Read the model definition and answer for the solid it produces. Units are mm, in the model's axes. Face numbers are marked on the shaded views. A direction names the side the tool comes from. Coordinates: 2 decimals unless noted, no trailing zeros. Write each loop counter-clockwise with the first axis right and the second up, starting at its lowest first coordinate (ties: lowest second). Pieces come first, ordered by that corner, then holes.
1) Determine the mould class of the marked faces 5, 6 and 7 for opening direction X: +X half, -X half, draft (parallel to the pull), parting line (faces both ways), or undercut.
2) Which of the six approach directions +Z, -Z, +X, -X, +Y, -Y give full straight-line access (tool end or side, diameter ignored) to the marked faces 1, 2, 3 and 4?
3) Each of these flat-tipped pins is pushed along its axis until it touches: pin 1 Ø5.5 at (x, z) = (-25.5, 12.5) entering from -Y; pin 2 Ø22.5 at (y, z) = (-8, 47) entering from -X; pin 3 Ø11.5 at (x, y) = (4.5, -1) entering from +Z; pin 4 Ø2 at (x, y) = (-9, 11) entering from -Z. Where does it stop, or does it pass through?
4) The part is cut by section C-C (z = 41.5). Determine the outline of the cut face in (x, y).
5) Find the intervals of material crossed by line 1 (X direction, y = 0, z = 6.25); line 2 (X direction, y = 7, z = 54); line 3 (Y direction, x = -57, z = 11), in increasing order.
6) The part is cut by section A-A (x = -57). Determine the outline of the cut face in (y, z), then the cut area to 3 significant figures.
7) The part is cut by section B-B (y = 0). Determine the outline of the cut face in (x, z), then the cut area to 3 significant figures.
8) The part is cut by section D-D (y = 25). Determine the outline of the cut face in (x, z), then the cut area to 3 significant figures.
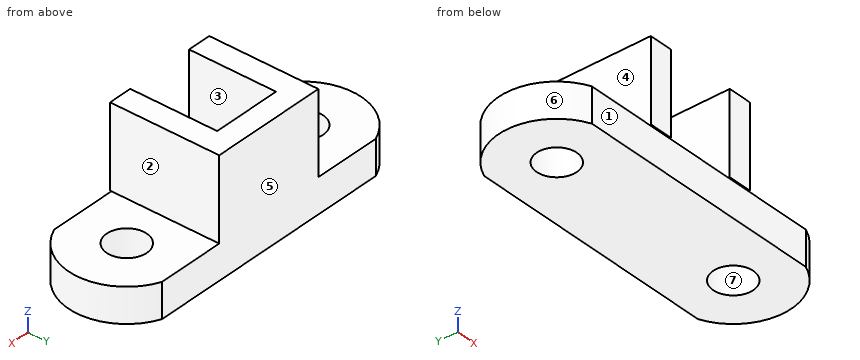
Autodesk Fusion 360 part; units mm, degrees
sketch "Sketch2" plane through (0, 0, 0) normal (0, 0, 1) x (1, 0, 0)
  line L0 (57, 29.6362) -> (-57, 29.6362)
  line L1 (-57, 29.6362) -> (-57, -29.6362)
  line L2 (-57, -29.6362) -> (57, -29.6362)
  line L3 (57, -29.6362) -> (57, 29.6362)
  line L4 (57, 29.6362) -> (-57, -29.6362) construction
  line L5 (-57, 29.6362) -> (57, -29.6362) construction
  circle A0 centre (57, 0) radius 11
  circle A1 centre (-57, 0) radius 11
  line L6 (57, 29.6362) -> (69.0705, 29.6362)
  line L7 (57, -29.6362) -> (69.0705, -29.6362)
  line L8 (69.0705, 29.6362) -> (69.0705, -29.6362)
  line L9 (-57, -29.6362) -> (-69.0705, -29.6362)
  line L10 (-57, 29.6362) -> (-69.0705, 29.6362)
  line L11 (-69.0705, 29.6362) -> (-69.0705, -29.6362)
  arc A2 (-69.0705, 29.6362) -> (-69.0705, -29.6362) centre (-57, 0) ccw
  arc A3 (69.0705, -29.6362) -> (69.0705, 29.6362) centre (57, 0) ccw
  dimension "d1" = 114
  dimension "d2" = 59.2723
  dimension "d3" = 22
  dimension "d4" = 22
  dimension "d5" = 64
  dimension "d6" = 64
extrude "Extrude1" add sketch "Sketch2" along normal blind 19 contours L0 L1 L2 L3 A0 A1 | L3 A0 L6 L7 L8 | L1 A1 L9 L10 L11 | L8 A3 | L11 A2
sketch "Sketch3" plane through (0, 0, 19) normal (0, 0, 1) x (-1, 0, 0)
  circle A0 centre (57, 0) radius 11
  circle A1 centre (-57, 0) radius 11
  line L0 (69.0705, 29.6362) -> (-69.0705, 29.6362)
  arc A2 (-69.0705, 29.6362) -> (-69.0705, -29.6362) centre (-57, 0) ccw
  line L1 (-69.0705, -29.6362) -> (69.0705, -29.6362)
  arc A3 (69.0705, -29.6362) -> (69.0705, 29.6362) centre (57, 0) ccw
  line L2 (32, -29.6362) -> (32, 29.6362) construction
  line L3 (-32, -29.6362) -> (-32, 29.6362) construction
  dimension "d9" = 64
  dimension "d10" = 25
sketch "Sketch4" plane through (0, 29.6362, 0) normal (0, 1, 0) x (-1, 0, 0)
  line L0 (-69.0705, 0) -> (69.0705, 0)
  line L1 (69.0705, 0) -> (69.0705, 19)
  line L2 (69.0705, 19) -> (-69.0705, 19)
  line L3 (-69.0705, 19) -> (-69.0705, 0)
  line L4 (-32.0857, 19) -> (31.9143, 19)
  line L5 (31.9143, 19) -> (31.9143, 64)
  line L6 (31.9143, 64) -> (-32.0857, 64)
  line L7 (-32.0857, 64) -> (-32.0857, 19)
  dimension "d11" = 64
  dimension "d12" = 45
extrude "Extrude2" add sketch "Sketch4" against normal blind 60 contours L2 L4 L5 L6 L7
sketch "Sketch5" plane through (0, 0, 64) normal (0, 0, 1) x (-1, 0, 0)
  line L0 (-32.0857, -29.6362) -> (31.9143, -29.6362)
  line L1 (31.9143, -29.6362) -> (31.9143, 30.3638)
  line L2 (31.9143, 30.3638) -> (-32.0857, 30.3638)
  line L3 (-32.0857, 30.3638) -> (-32.0857, -29.6362)
  line L4 (31.9143, -17.4462) -> (-32.0857, -17.4462)
  line L5 (18.9143, -17.4462) -> (18.9143, 30.3638)
  line L6 (-19.0857, -17.4462) -> (-19.0857, 30.3638)
  dimension "d15" = 12.19
  dimension "d16" = 38
  dimension "d17" = 13
extrude "Extrude3" cut sketch "Sketch5" against normal blind 45 contours L2 L4 L5 L6
equation "d12 = 64 mm - 19 mm"
Reported:
1. face 5: draft
1. face 6: -X half
1. face 7: undercut
2. face 1: -Z, +X, -X, -Y
2. face 2: +Z, +X, +Y, -Y
2. face 3: +Z, -Y
2. face 4: +Z, -X, +Y, -Y
3. pin 1: stops at y = -29.64
3. pin 2: stops at x = -31.91
3. pin 3: stops at z = 19
3. pin 4: stops at z = 0
4. outline: (-31.91, -30.36) - (-18.91, -30.36) - (-18.91, 17.45) - (19.09, 17.45) - (19.09, -30.36) - (32.09, -30.36) - (32.09, 29.64) - (-31.91, 29.64) - close
5. line 1: x = -89 to -68, -46 to 46, 68 to 89
5. line 2: x = -31.91 to -18.91, 19.09 to 32.09
5. line 3: y = -29.64 to -11, 11 to 29.64
6. outline: (-29.64, 0) - (-11, 0) - (-11, 19) - (-29.64, 19) - close; (11, 0) - (29.64, 0) - (29.64, 19) - (11, 19) - close
6. area: 708 mm2
7. outline: (-89, 0) - (-68, 0) - (-68, 19) - (-89, 19) - close; (-46, 0) - (46, 0) - (46, 19) - (32.09, 19) - (32.09, 64) - (19.09, 64) - (19.09, 19) - (-18.91, 19) - (-18.91, 64) - (-31.91, 64) - (-31.91, 19) - (-46, 19) - close; (68, 0) - (89, 0) - (89, 19) - (68, 19) - close
7. area: 3,720 mm2
8. outline: (-76.98, 0) - (76.98, 0) - (76.98, 19) - (32.09, 19) - (32.09, 64) - (-31.91, 64) - (-31.91, 19) - (-76.98, 19) - close
8. area: 5,810 mm2
